The model under review builds one solid part; all positions refer to its coordinate system, in mm. Give positions to 0.01 mm unless a question says otherwise; leave off trailing zeros. Loops run counter-clockwise (first coordinate to the right, second up) from the corner with the lowest first, then second, coordinate; pieces in that order, holes last. Notation, with made-up numbers: M 6.25,31.25 L 25.25,31.25 A27 ccw 25.25,49.25 Z; hole C 2.5,-39 d9. An arc over 180 degrees is marked long. Return JSON: item names as keys, results as strings.
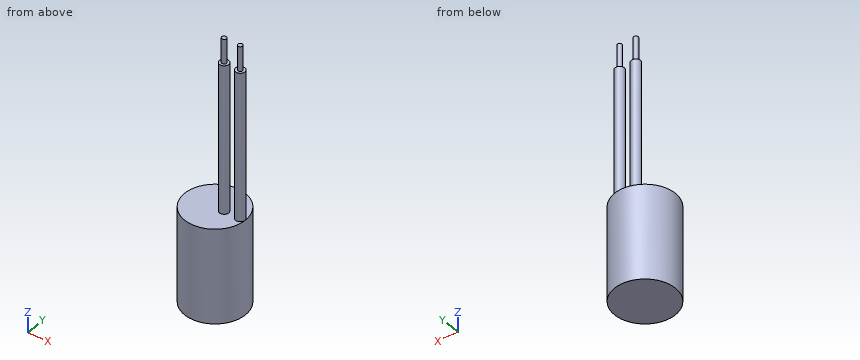
```python
from build123d import *

# Parameters (mm, degrees)
F0_R     = 23.495
F1_DEPTH = 73.152
F2_R     = 3.6195
F3_DEPTH = 114.554
F4_R     = 1.778
F5_DEPTH = 19.05


with BuildPart() as f1:
    # F0 (on Top) → F1 (new body)
    with BuildSketch(Plane.XY):
        Circle(F0_R)
    extrude(amount=F1_DEPTH)

    # F2 (on face) → F3 (join)
    with BuildSketch(Plane.XY.offset(73.152)):
        with Locations((19.812, 0)):
            Circle(F2_R)
        with Locations((7.112, 0)):
            Circle(F2_R)
    extrude(amount=F3_DEPTH)

    # F4 (on face) → F5 (join)
    with BuildSketch(Plane.XY.offset(187.706)):
        with Locations((7.112, 0)):
            Circle(F4_R)
        with Locations((19.812, 0)):
            Circle(F4_R)
    extrude(amount=F5_DEPTH)


solid = f1.part
```
1) Consider section A-A on z = 135.5. Write out the cut boundary in (x, y), then the cut area to 3 significant figures.
From the geometry:
{"outline": "C 7.11,0 d7.24; C 19.81,0 d7.24", "area": "82.3 mm²"}
2) Consider section B-B on z = 40. Write out the cut boundary in (x, y) (3 decimals).
From the geometry:
{"outline": "C 0,0 d46.99"}
3) Wall thickness on L1, parallel to Z at x = -15.5, y = -17; L2, parallel to X at y = -3, z = 131; L3, parallel to Y at x = 19.5, z = 131: over which ranges is each line inside the solid? List them lowest first. Write a range as from..to.
From the geometry:
{"L1": "0..73.15", "L2": "5.09..9.14, 17.79..21.84", "L3": "-3.61..3.61"}
4) Consider section C-C on x = -13.5. Write out the cut boundary in (y, z), then the cut area to 3 significant figures.
From the geometry:
{"outline": "M -19.23,0 L 19.23,0 L 19.23,73.15 L -19.23,73.15 Z", "area": "2,810 mm²"}
5) Insertion check: pin 1 (5 mm diameter, centred on x = 11.5, z = 64, fed in from -Y); pin 2 (2 mm diameter, centred on x = 1.5, y = -11.5, fed in from +Z); pin 3 (4 mm diameter, centred on y = 0.5, z = 111.5, fed in from -X). Each pin has a flat end and moves straight along its axis. Give the tip position at first contact, or say it passes through.
From the geometry:
{"pin 1": "y = -21.7", "pin 2": "z = 73.15", "pin 3": "x = 3.49"}
6) Consider section D-D on y = 7. Write out the cut boundary in (x, z).
From the geometry:
{"outline": "M -22.43,0 L 22.43,0 L 22.43,73.15 L -22.43,73.15 Z"}
